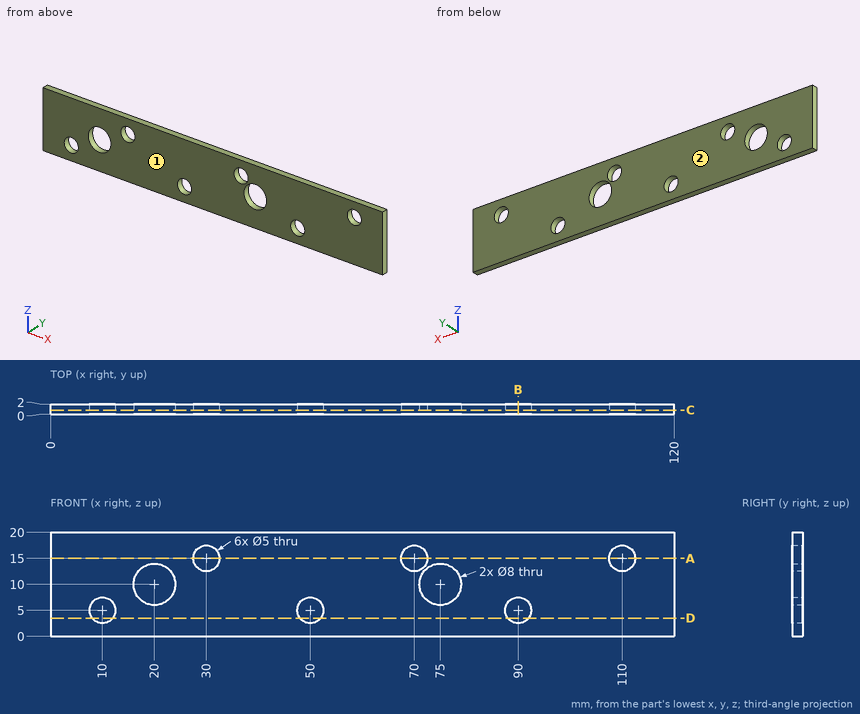
Job drawing, mm, ordinate dimensions from the low corner. One solid piece. Coordinates: 2 decimals unless noted, no trailing zeros. Write each loop counter-clockwise with the first axis right and the second up, starting at its lowest first coordinate (ties: lowest second). Pieces come first, ordered by that corner, then holes. Notation, with made-up numbers: (85.5, 13.25) - (138.5, 13.25) arc R21 cw to (138.5, 32.25) - close; hole circle Ø8 at (-24, 32). An arc over 180 degrees is marked (long way). Use a Markdown table: item, result. Add a question column.
Item 1: Flat gauge pin, fed straight in: pin 1 (4 mm diameter, centred on x = 30, z = 15, fed in from +Y). Where does the tip first touch, or does it go through?
Item 2: Band-saw the part on C-C, the plane y = 0.8. Give the number of separate pieces and of enclosed holes in the cut face, and give its area (3 significant figures).
Item 3: Band-saw the part on A-A, the plane z = 15. Give the cut face in (x, y), and give its area (3 significant figures).
Item 4: Band-saw the part on B-B, the plane x = 90. Give the cut face in (y, z), and give its area (3 significant figures).
Item 5: Band-saw the part on D-D, the plane z = 3.5. Give the cut face in (x, y).
Item 6: Drill centre lines: L1, parallel to X at y = 0.9, z = 5; L2, parallel to X at y = 0.9, z = 10; L3, parallel to X at y = 0.4, z = 15. Where is each one in solid material? Low to high. Write a range as from..to.
Item 7: Mould opens along Y. For the marked faces 1 and 2 say: pulls with the +Y half, pulls with the -Y half, needs draft (parallel to the pull), parting line crosses it, or undercut.
Numbers:
| question | item | result |
|---|---|---|
| 1 | pin 1 | through |
| 2 | separate pieces | 1 |
| 2 | enclosed holes | 8 |
| 2 | area | 2,180 mm2 |
| 3 | outline | (0, 0) - (27.5, 0) - (27.5, 2) - (0, 2) - close; (32.5, 0) - (67.5, 0) - (67.5, 2) - (32.5, 2) - close; (72.5, 0) - (107.5, 0) - (107.5, 2) - (72.5, 2) - close; (112.5, 0) - (120, 0) - (120, 2) - (112.5, 2) - close |
| 3 | area | 210 mm2 |
| 4 | outline | (0, 0) - (2, 0) - (2, 2.5) - (0, 2.5) - close; (0, 7.5) - (2, 7.5) - (2, 20) - (0, 20) - close |
| 4 | area | 30.0 mm2 |
| 5 | outline | (0, 0) - (8, 0) - (8, 2) - (0, 2) - close; (12, 0) - (48, 0) - (48, 2) - (12, 2) - close; (52, 0) - (88, 0) - (88, 2) - (52, 2) - close; (92, 0) - (120, 0) - (120, 2) - (92, 2) - close |
| 6 | L1 | 0..7.5, 12.5..47.5, 52.5..87.5, 92.5..120 |
| 6 | L2 | 0..16, 24..71, 79..120 |
| 6 | L3 | 0..27.5, 32.5..67.5, 72.5..107.5, 112.5..120 |
| 7 | face 1 | pulls with the -Y half |
| 7 | face 2 | pulls with the +Y half |
